Source: CAD feature listing. Evaluate the final solid. Frame: model axes, mm. A direction names the side the tool comes from. Coordinates: 2 decimals unless noted, no trailing zeros. Order: outer loops, then holes, each group sorted by start corner. A loop starts at its lowest first (then second) coordinate and runs counter-clockwise, first axis right, second up.
```python
from build123d import *

# Parameters (mm, degrees)
PAD_DEPTH       = 50
SKETCH001_R     = 2.15
POCKET_DEPTH    = 5
SKETCH002_R     = 3.3
POCKET001_DEPTH = 5
SKETCH003_R     = 3.3
POCKET002_DEPTH = 5


with BuildPart() as part:
    # Sketch → Pad (new body)
    with BuildSketch(Plane.XY):
        Polygon((0, 26), (0, 0), (19.9512810052, 1.3951294749), (20.1605504264, -1.5975626759), (-3, -3.2171061301), (-43, -3.2171061301), (-43, -0.2171061301), (-3, -0.2171061301), (-3, 29.2171061301), (20.1605504264, 27.5975626759), (19.9512810052, 24.6048705251), align=None)
    extrude(amount=PAD_DEPTH)

    # Sketch001 (on Face7 of Pad) → Pocket (cut)
    with BuildSketch(Plane(origin=(0, -0.2171061301, 0), x_dir=(-1, 0, 0), z_dir=(0, 1, 0))):
        with Locations((13, 45)):
            Circle(SKETCH001_R)
        with Locations((33, 45)):
            Circle(SKETCH001_R)
        with Locations((13, 5)):
            Circle(SKETCH001_R)
        with Locations((33, 5)):
            Circle(SKETCH001_R)
    extrude(amount=-POCKET_DEPTH, mode=Mode.SUBTRACT)

    # Sketch002 (on Face13 of Pocket) → Pocket001 (cut)
    with BuildSketch(Plane(origin=(2.0185197337, 28.8661770444, 0), x_dir=(-0.9975640503, 0.0697564737, 0), z_dir=(0.0697564737, 0.9975640503, 0))):
        with Locations((-5.9692255526, 25)):
            Circle(SKETCH002_R)
    extrude(amount=-POCKET001_DEPTH, mode=Mode.SUBTRACT)

    # Sketch003 (on Face3 of Pocket001) → Pocket002 (cut)
    with BuildSketch(Plane(origin=(0, 0, 0), x_dir=(-0.9975640503, -0.0697564737, 0), z_dir=(-0.0697564737, 0.9975640503, 0))):
        with Locations((-11, 25)):
            Circle(SKETCH003_R)
    extrude(amount=-POCKET002_DEPTH, mode=Mode.SUBTRACT)


solid = part.part
```
Q1. Section query D-D on x = -34. Output: boundary loops of the cut face in (y, z).
Solutions:
outline: (-3.22, 0) - (-0.22, 0) - (-0.22, 3.1) - (-3.22, 3.1) - close; (-3.22, 6.9) - (-0.22, 6.9) - (-0.22, 43.1) - (-3.22, 43.1) - close; (-3.22, 46.9) - (-0.22, 46.9) - (-0.22, 50) - (-3.22, 50) - close
Q2. Pull-direction query (Y, two-part tool) for faces 6 (the cylindrical face through (6.351, 27.081, 22.072)), 7 (the flat face through (-43, -2, 25)), 8 (the flat face through (13.56, 28.06, 24.65)); classes: pulls with the +Y half, pulls with the -Y half, needs draft (parallel to the pull), parting line crosses it, or undercut.
Solutions:
face 6: undercut
face 7: needs draft
face 8: pulls with the +Y half
Q3. Section query C-C on z = 8.5. Output: boundary loops of the cut face in (x, y), plus the area to 3 significant figures.
Solutions:
outline: (-43, -3.22) - (-3, -3.22) - (20.16, -1.6) - (19.95, 1.4) - (0, 0) - (0, 26) - (19.95, 24.6) - (20.16, 27.6) - (-3, 29.22) - (-3, -0.22) - (-43, -0.22) - close
area: 337 mm2
Q4. Material intervals for line 1 along Z through (x, y) = (-33, -1.55); line 2 along X through (y, z) = (5, 3.5); line 3 along Y through (x, z) = (-28, 7), sorted ascending.
Solutions:
line 1: z = 0 to 2.85, 7.15 to 42.85, 47.15 to 50
line 2: x = -3 to 0
line 3: y = -3.22 to -0.22
Q5. Section query A-A on x = -13. Output: boundary loops of the cut face in (y, z).
Solutions:
outline: (-3.22, 0) - (-0.22, 0) - (-0.22, 2.85) - (-3.22, 2.85) - close; (-3.22, 7.15) - (-0.22, 7.15) - (-0.22, 42.85) - (-3.22, 42.85) - close; (-3.22, 47.15) - (-0.22, 47.15) - (-0.22, 50) - (-3.22, 50) - close
Q6. Section query B-B on z = 27. Output: boundary loops of the cut face in (x, y).
Solutions:
outline: (-43, -3.22) - (-3, -3.22) - (8.56, -2.41) - (8.35, 0.58) - (0, 0) - (0, 26) - (5.15, 25.64) - (5.35, 28.63) - (-3, 29.22) - (-3, -0.22) - (-43, -0.22) - close; (10.38, 25.27) - (19.95, 24.6) - (20.16, 27.6) - (10.59, 28.27) - close; (13.59, 0.95) - (13.8, -2.04) - (20.16, -1.6) - (19.95, 1.4) - close
Q7. Pin query (flat end, axial travel): P1, Ø3, axis at y = 12.5, z = 28, coming from the +X side; P2, Ø5, axis at x = 7, z = 32, coming from the -Y side; P3, Ø14.5, axis at y = 16.5, z = 22.5, coming from the -X side. Return the tip coordinate at first contact, or that it passes through.
Solutions:
P1: stops at x = 0
P2: stops at y = -2.69
P3: stops at x = -3
Q8. Set-up query: faces 1 (the flat face through (12.332, 25.138, 24.65)), 2 (the cylindrical face through (-14.16, -1.7, 46.81)), 3 (the flat face through (-2, 8, 0)), 4 (the flat face through (-23, -0.217, 25)), 5 (the flat face through (20.057, 26.122, 24.65)). Return all of +Z, -Z, +X, -X, +Y, -Y with unobstructed straight access to the full face (end or side cutting, diameter ignored); none if empty.
Solutions:
face 1: +Z, -Z
face 2: +Y, -Y
face 3: -Z, +X, -X, +Y, -Y
face 4: +Z, -Z, -X, +Y
face 5: +Z, -Z, +X
